```python
from build123d import *

# Parameters (mm, degrees)
SKETCH1_W           = 25.5
SKETCH1_H           = 35
BOSS_EXTRUDE1_DEPTH = 1.5875
SKETCH2_W           = 15.116457136
SKETCH2_H           = 15.832029072
BOSS_EXTRUDE2_DEPTH = 4.9125
CUT_EXTRUDE1_REACH  = 24.202
SKETCH3_R           = 1.122559654


with BuildPart() as part:
    # Sketch1 → Boss-Extrude1 (new body)
    with BuildSketch(Plane(origin=(0, 0, 0), x_dir=(1, 0, 0), z_dir=(0, 1, 0))):
        Rectangle(SKETCH1_W, SKETCH1_H)
    extrude(amount=BOSS_EXTRUDE1_DEPTH)

    # Sketch2 → Boss-Extrude2 (add)
    with BuildSketch(Plane(origin=(0, 1.5875, 0), x_dir=(1, 0, 0), z_dir=(0, 1, 0))):
        with Locations((-0.983911411, 0.380147591)):
            Rectangle(SKETCH2_W, SKETCH2_H)
    extrude(amount=BOSS_EXTRUDE2_DEPTH)

    # Sketch3 → Cut-Extrude1 (cut, up to next)
    with BuildSketch(Plane(origin=(0, 1.5875, 0), x_dir=(1, 0, 0), z_dir=(0, 1, 0)), mode=Mode.PRIVATE) as cut_extrude1_sk1:
        with Locations(Location((-10.110032203, 14.949417208, 0), (0, 0, 270))):
            Circle(SKETCH3_R)
    cut_extrude1_tool1 = extrude(cut_extrude1_sk1.sketch, amount=-CUT_EXTRUDE1_REACH, mode=Mode.PRIVATE) & part.part
    # Sketch3 → Cut-Extrude1 (cut, up to next)
    with BuildSketch(Plane(origin=(0, 1.5875, 0), x_dir=(1, 0, 0), z_dir=(0, 1, 0)), mode=Mode.PRIVATE) as cut_extrude1_sk2:
        with Locations(Location((10.110032203, 14.949417208, 0), (0, 0, 270))):
            Circle(SKETCH3_R)
    cut_extrude1_tool2 = extrude(cut_extrude1_sk2.sketch, amount=-CUT_EXTRUDE1_REACH, mode=Mode.PRIVATE) & part.part
    add(cut_extrude1_tool1.solids().sort_by_distance((-10.110032, 1.5875, -14.949417))[0], mode=Mode.SUBTRACT)
    add(cut_extrude1_tool2.solids().sort_by_distance((10.110032, 1.5875, -14.949417))[0], mode=Mode.SUBTRACT)


solid = part.part
```
Geometry check sheet. Reference: the model listing, model coordinates, mm. A direction names the side the tool comes from. Coordinates: 2 decimals unless noted, no trailing zeros. Order: outer loops, then holes, each group sorted by start corner. A loop starts at its lowest first (then second) coordinate and runs counter-clockwise, first axis right, second up. Notation, with made-up numbers: (82, -9) - (120, -9) arc R25 ccw to (120, 10) - close; hole circle Ø6 at (53.25, -9). An arc over 180 degrees is marked (long way). Answer in a Markdown table with one row per item. Add a question column.
1. Section check D-D (y = 4). Enter the section's corners in (x, z).
2. Section check B-B (x = -10.75). Enter the section's corners in (y, z).
3. Gauge pin test, flat ends, axial feed: pin 1 Ø1.5 at (x, y) = (1, 3) entering from -Z; pin 2 Ø2.5 at (y, z) = (4.5, 1) entering from -X; pin 3 Ø1.3 at (x, z) = (10.11, -14.95) entering from +Y; pin 4 Ø2.5 at (y, z) = (5, 0) entering from +X. Record the tip position at first contact, or that the pin passes through.
4. Access from +Z, -Z, +X, -X, +Y, -Y to the whole of each face (thin tool, end or side, straight path). Record for faces 1 (the face through (-1, 4, 7.536)), 2 (the face through (-8.542, 4, 0)), 3 (the face through (6.574, 4, 0)).
5. Section check A-A (z = -4). Enter the section's corners in (x, y).
6. Section check C-C (x = 1.75). Enter the section's corners in (y, z), plus the area to 3 significant figures.
7. Material ranges on L1, parallel to Y at x = 9.5, z = 10.5; L2, parallel to X at y = 2.5, z = 5.5; L3, parallel to Z at x = 4.75, y = 2.25, recorded low to high. Write a range as [from, to].
8. Draft check along Z on faces 4 (the face through (-8.997, 0.805, -15.096)), 5 (the face through (-12.75, 1, 0)), 6 (the face through (-1, 4, -8.296)). Enter one of: +Z half, -Z half, draft (parallel to the pull), parting line (faces both ways), or undercut.
Data:
| question | item | result |
|---|---|---|
| 1 | outline | (-8.54, -8.3) - (6.57, -8.3) - (6.57, 7.54) - (-8.54, 7.54) - close |
| 2 | outline | (0, -17.5) - (1.59, -17.5) - (1.59, -15.87) - (0, -15.87) - close; (0, -14.03) - (1.59, -14.03) - (1.59, 17.5) - (0, 17.5) - close |
| 3 | pin 1 | stops at z = -8.3 |
| 3 | pin 2 | stops at x = -8.54 |
| 3 | pin 3 | passes through |
| 3 | pin 4 | stops at x = 6.57 |
| 4 | face 1 | +Z, +X, -X, +Y |
| 4 | face 2 | +Z, -Z, -X, +Y |
| 4 | face 3 | +Z, -Z, +X, +Y |
| 5 | outline | (-12.75, 0) - (12.75, 0) - (12.75, 1.59) - (6.57, 1.59) - (6.57, 6.5) - (-8.54, 6.5) - (-8.54, 1.59) - (-12.75, 1.59) - close |
| 6 | outline | (0, -17.5) - (1.59, -17.5) - (1.59, -8.3) - (6.5, -8.3) - (6.5, 7.54) - (1.59, 7.54) - (1.59, 17.5) - (0, 17.5) - close |
| 6 | area | 133 mm² |
| 7 | L1 | y = [0, 1.59] |
| 7 | L2 | x = [-8.54, 6.57] |
| 7 | L3 | z = [-8.3, 7.54] |
| 8 | face 4 | undercut |
| 8 | face 5 | draft |
| 8 | face 6 | -Z half |
